Geometry: final body of the model. Coordinates: model frame, mm. A direction names the side the tool comes from. Give positions to 0.01 mm unless a question says otherwise; leave off trailing zeros. Write each loop counter-clockwise with the first axis right and the second up, starting at its lowest first coordinate (ties: lowest second). Pieces come first, ordered by that corner, then holes. Notation, with made-up numbers: M 85.5,-21 L 136.5,-21 A14 ccw 136.5,-14 Z; hole C -38.75,35 d9. An arc over 180 degrees is marked long. Use one line per item in the form item = value. Start each with the question number.
Item 1: Pull-direction query (Y, two-part tool) for faces 3 (the flat face through (5, 6.77, 9)), 4 (the flat face through (124, 15, 14.56)), 5 (the cylindrical face through (224.884, 11.524, 8.368)); classes: released by +Y, released by -Y, zero draft, split by the parting line, or undercut.
Item 2: Access query for faces 1 (the flat face through (247, 3, 2.81)), 2 (the flat face through (124, 11, 0)). Directions: +Z, -Z, +X, -X, +Y, -Y. A direction counts if a zero-diameter tool reaches every point of the face in a straight line with its end or side. Return the directions, or none.
Item 3: Section query A-A on x = 222.79. Return loops of the section in (y, z), then the cut area to 3 significant figures.
Item 4: Contact query for flat-ended pins moving along their axis: P1, Ø4, axis at y = 6.5, z = 7.5, coming from the -X side; P2, Ø1.4, axis at y = 3.5, z = 1, coming from the +X side; P3, Ø4, axis at x = 110.5, z = 5, coming from the -Y side; P4, Ø5.5, axis at x = 222.79, y = 10.865, coming from the -Z side. Output: stop coordinate, or through.
Item 5: Section query B-B on x = 76.5. Return loops of the section in (y, z).
Item 6: Section query C-C on z = 12.5. Return loops of the section in (x, y) (3 decimals), then the cut area to 3 significant figures.
Item 7: Material intervals for line 1 along X through (y, z) = (3.5, 2); line 2 along X through (y, z) = (10.75, 12.75); line 3 along X through (y, z) = (18.25, 1.75), sorted ascending. Write a range as from..to.
from build123d import *

# Parameters (mm, degrees)
BOX001_W        = 251.83
BOX001_H        = 6.77
BOX001_DEPTH    = 11.75
BOX_W           = 251.83
BOX_H           = 22.03
BOX_DEPTH       = 14.56
SKETCH_R        = 2.195
POCKET_DEPTH    = 14.561
POCKET001_DEPTH = 14.561
FILLET_R        = 2
FILLET001_R     = 2
FILLET002_R     = 2


with BuildPart() as cubo001:
    # Box001 → Box001 (new body)
    with BuildSketch(Plane.XY.offset(2.81)):
        with Locations((125.915, 3.385)):
            Rectangle(BOX001_W, BOX001_H)
    extrude(amount=BOX001_DEPTH)


with BuildPart() as fillet002:
    # Box → Box (new body)
    with BuildSketch(Plane.XY):
        with Locations((125.915, 11.015)):
            Rectangle(BOX_W, BOX_H)
    extrude(amount=BOX_DEPTH)

    # Cut: cut Cubo001
    add(cubo001.part, mode=Mode.SUBTRACT)

    # Sketch (on Face5 of Cut) → Pocket (cut, through all)
    with BuildSketch(Plane.XY.offset(14.56)):
        with Locations((27.795, 10.865)):
            Circle(SKETCH_R)
        with Locations((222.79, 10.865)):
            Circle(SKETCH_R)
    extrude(amount=-POCKET_DEPTH, mode=Mode.SUBTRACT)

    # Sketch001 (on Face7 of Pocket) → Pocket001 (cut, through all)
    with BuildSketch(Plane(origin=(0, 0, 0), x_dir=(1, 0, 0), z_dir=(0, 0, -1))):
        with BuildLine():
            Line((10.048096, -5.5), (10.048096, -2.5))
            ThreePointArc((10.048096, -2.5), (10.333563, -1.247868), (10.03, 0))
            Line((17.21, 0), (10.03, 0))
            ThreePointArc((17.21, 0), (16.906437, -1.247868), (17.191904, -2.5))
            Line((17.191904, -5.5), (17.191904, -2.5))
            ThreePointArc((10.048096, -5.5), (13.62, -8.73), (17.191904, -5.5))
        make_face()
        with BuildLine():
            ThreePointArc((234.62, -5.14), (238.21, -8.73), (241.8, -5.14))
            Line((241.8, -5.14), (241.8, -2.14))
            ThreePointArc((241.8, 0), (241.587489, -1.07), (241.8, -2.14))
            Line((241.8, 0), (234.62, 0))
            ThreePointArc((234.62, -2.14), (234.832511, -1.07), (234.62, 0))
            Line((234.62, -2.14), (234.62, -5.14))
        make_face()
    extrude(amount=-POCKET001_DEPTH, mode=Mode.SUBTRACT)

    # Fillet
    fillet_edges = [fillet002.edges().sort_by_distance(p)[0] for p in [
        (0, 0, 1.405),
        (0, 22.03, 7.28),
        (251.83, 22.03, 7.28),
        (251.83, 0, 1.405),
    ]]
    fillet(fillet_edges, radius=FILLET_R)

    # Fillet001
    fillet001_edges = [fillet002.edges().sort_by_distance(p)[0] for p in [
        (220.595, 10.865, 0),
        (25.6, 10.865, 0),
    ]]
    fillet(fillet001_edges, radius=FILLET001_R)

    # Fillet002
    fillet002_edges = [fillet002.edges().sort_by_distance(p)[0] for p in [
        (125.915, 22.03, 0),
        (0, 11.015, 0),
        (251.83, 11.015, 0),
        (6.015, 0, 0),
        (245.815, 0, 0),
        (125.915, 0, 0),
    ]]
    fillet(fillet002_edges, radius=FILLET002_R)


solid = fillet002.part
Answer sheet:
q1.face_3 = released by -Y
q1.face_4 = zero draft
q1.face_5 = undercut
q2.face_1 = +Z, +X, -X, -Y
q2.face_2 = -Z, +X, -X, +Y, -Y
q3.outline = M 0,2 A2 ccw 2,0 L 6.67,0 A2 ccw 8.67,2 L 8.67,14.56 L 6.77,14.56 L 6.77,2.81 L 0,2.81 Z; M 13.06,2 A2 ccw 15.06,0 L 20.03,0 A2 ccw 22.03,2 L 22.03,14.56 L 13.06,14.56 Z
q3.area = 174 mm2
q4.P1 = 0
q4.P2 = 251.81
q4.P3 = 6.77
q4.P4 = 0.62
q5.outline = M 0,2 A2 ccw 2,0 L 20.03,0 A2 ccw 22.03,2 L 22.03,14.56 L 6.77,14.56 L 6.77,2.81 L 0,2.81 Z
q6.outline = M 0,6.77 L 10.421,6.77 A3.59 cw 16.819,6.77 L 235.011,6.77 A3.59 cw 241.409,6.77 L 251.83,6.77 L 251.83,20.03 A2 ccw 249.83,22.03 L 2,22.03 A2 ccw 0,20.03 Z; hole C 27.795,10.865 d4.39; hole C 222.79,10.865 d4.39
q6.area = 3,790 mm2
q7.line_1 = 0..10.05, 17.19..234.62, 241.8..251.83
q7.line_2 = 0..25.6, 29.99..220.6, 224.98..251.83
q7.line_3 = 0.02..251.81
